Input: part model. Units: mm. Frame: model coordinates. Face numbers are marked on the shaded views. A direction names the side the tool comes from. Round coordinates to 2 decimals unless told otherwise and drop trailing zeros. Loops run counter-clockwise (first coordinate to the right, second up) from the corner with the lowest first, then second, coordinate; pieces in that order, holes last. Notation, with made-up numbers: M -3,3 L 46,3 A11 ccw 46,19 Z; hole C -35,58 d3. An arc over 180 degrees is marked long. Return JSON: item names as keys, results as strings. Group by question number.
1) Access query for the marked faces 1, 2, 3, 4 and 5. Directions: +Z, -Z, +X, -X, +Y, -Y. A direction counts if a zero-diameter tool reaches every point of the face in a straight line with its end or side. Return the directions, or none.
2) Contact query for flat-ended pins moving along their axis: P1, Ø1, axis at y = 11, z = 55, coming from the +X side; P2, Ø14, axis at x = 61.5, z = 40.5, coming from the +Y side; P3, Ø6, axis at x = -3.5, z = 52.5, coming from the -Y side. Output: stop coordinate, or through.
3) Section D-D (y = 37). Output: boundary loops of the cut face in (x, z).
4) Mould query, pull axis Z, two halves, no side actions, for the marked faces 6, 7, 8 and 9. Classes: +Z half, -Z half, draft (parallel to the pull), parting line (faces both ways), or undercut.
5) Section C-C (x = -2.5). Output: boundary loops of the cut face in (y, z).
6) Material intervals for line 1 (X direction, y = 12, z = 53); line 2 (Y direction, x = -45, z = 59); line 3 (Z direction, x = 63, y = 21.5), sorted ascending. Write a range as from..to.
7) Section A-A (z = 75.5). Output: boundary loops of the cut face in (x, y), plus the area to 3 significant figures.
8) Section B-B (x = 45). Output: boundary loops of the cut face in (y, z), plus the area to 3 significant figures.
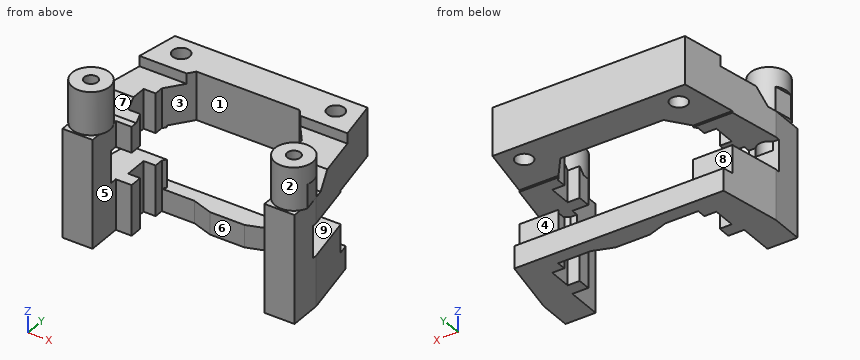
from build123d import *

# Parameters (mm, degrees)
SZKIC1_W                        = 1
SZKIC1_H                        = 32
DODANIE_WYCI_GNI_CIE1_DEPTH     = 67.5
WYTNIJ_WYCI_GNI_CIE1_DEPTH      = 94
WYTNIJ_WYCI_GNI_CIE2_DEPTH      = 36
WYTNIJ_WYCI_GNI_CIE2_DEPTH_BACK = 135
WYTNIJ_WYCI_GNI_CIE6_REACH      = 131.943
SZKIC6_R                        = 5
SZKIC7_R                        = 6.5
WYTNIJ_WYCI_GNI_CIE7_DEPTH      = 20
SZKIC8_R                        = 11
SZKIC8_R_2                      = 3.9
DODANIE_WYCI_GNI_CIE2_DEPTH     = 25
WYTNIJ_WYCI_GNI_CIE8_DEPTH      = 94


with BuildPart() as part:
    # Szkic1 → Dodanie-wyciągnięcie1 (new, symmetric)
    with BuildSketch(Plane(origin=(0, 0, 0), x_dir=(0, 0, -1), z_dir=(1, 0, 0))):
        Polygon((-63, 24), (-71, 32), (-71, 56), (-77, 56), (-77, 80), (-49, 80), (-49, 16), (-29.3, 16), (-29.3, 48), (-13, 48), (-13, 54), (0, 54), (0, 0), (-63, 0), align=None)
        with Locations((-48.5, 32)):
            Rectangle(SZKIC1_W, SZKIC1_H)
    extrude(amount=DODANIE_WYCI_GNI_CIE1_DEPTH, both=True)

    # Szkic2 → Wytnij-wyciągnięcie1 (cut)
    with BuildSketch(Plane(origin=(0, 0, 0), x_dir=(-1, 0, 0), z_dir=(0, 0, -1))):
        Polygon((50, 0), (50, 20), (40.75, 20), (40.75, 27.4), (47.75, 27.4), (47.75, 40.7), (40.75, 40.7), (40.75, 46), (21.75, 46), (10, 42), (-10, 42), (-21.75, 46), (-40.75, 46), (-40.75, 40.7), (-47.75, 40.7), (-47.75, 27.4), (-40.75, 27.4), (-40.75, 20), (-50, 20), (-50, 0), align=None)
    extrude(amount=-WYTNIJ_WYCI_GNI_CIE1_DEPTH, mode=Mode.SUBTRACT)

    # Szkic4 → Wytnij-wyciągnięcie2 (cut, two sides: drawn at the far end of the back side and taken through both)
    with BuildSketch(Plane(origin=(0, 0, 49), x_dir=(-1, 0, 0), z_dir=(0, 0, -1)).offset(-WYTNIJ_WYCI_GNI_CIE2_DEPTH_BACK)):
        Polygon((40.75, 40.7), (40.75, 46), (30, 60), (-30, 60), (-40.75, 46), (-40.75, 40.7), align=None)
    extrude(amount=WYTNIJ_WYCI_GNI_CIE2_DEPTH + WYTNIJ_WYCI_GNI_CIE2_DEPTH_BACK, mode=Mode.SUBTRACT)

    # Szkic6 → Wytnij-wyciągnięcie6 (cut, up to next)
    with BuildSketch(Plane.XY.offset(77), mode=Mode.PRIVATE) as wytnij_wyci_gni_cie6_sk1:
        with Locations((-45, 69)):
            Circle(SZKIC6_R)
    wytnij_wyci_gni_cie6_tool1 = extrude(wytnij_wyci_gni_cie6_sk1.sketch, amount=-WYTNIJ_WYCI_GNI_CIE6_REACH, mode=Mode.PRIVATE) & part.part
    # Szkic6 → Wytnij-wyciągnięcie6 (cut, up to next)
    with BuildSketch(Plane.XY.offset(77), mode=Mode.PRIVATE) as wytnij_wyci_gni_cie6_sk2:
        with Locations(Location((45, 69, 0), (0, 0, 270))):
            Circle(SZKIC6_R)
    wytnij_wyci_gni_cie6_tool2 = extrude(wytnij_wyci_gni_cie6_sk2.sketch, amount=-WYTNIJ_WYCI_GNI_CIE6_REACH, mode=Mode.PRIVATE) & part.part
    add(wytnij_wyci_gni_cie6_tool1.solids().sort_by_distance((-45, 69, 77))[0], mode=Mode.SUBTRACT)
    add(wytnij_wyci_gni_cie6_tool2.solids().sort_by_distance((45, 69, 77))[0], mode=Mode.SUBTRACT)

    # Szkic7 → Wytnij-wyciągnięcie7 (cut)
    with BuildSketch(Plane.XY.offset(63)):
        with Locations((-59, 12)):
            Circle(SZKIC7_R)
        with Locations(Location((59, 12, 0), (0, 0, 37.979872445))):
            Circle(SZKIC7_R)
    extrude(amount=-WYTNIJ_WYCI_GNI_CIE7_DEPTH, mode=Mode.SUBTRACT)

    # Szkic8 → Dodanie-wyciągnięcie2 (add)
    # profile 1 of 2: a face of its own
    with BuildSketch(Plane.XY.offset(63)):
        with Locations(Location((-59, 12, 0), (0, 0, 219.400568754))):
            Circle(SZKIC8_R)
        with Locations((-59, 12)):
            Circle(SZKIC8_R_2, mode=Mode.SUBTRACT)
    # profile 2 of 2: a face of its own
    with BuildSketch(Plane.XY.offset(63)):
        with Locations(Location((59, 12, 0), (0, 0, 180))):
            Circle(SZKIC8_R)
        with Locations(Location((59, 12, 0), (0, 0, 180))):
            Circle(SZKIC8_R_2, mode=Mode.SUBTRACT)
    extrude(amount=DODANIE_WYCI_GNI_CIE2_DEPTH)

    # Szkic9 → Wytnij-wyciągnięcie8 (cut)
    with BuildSketch(Plane.XY.offset(77)):
        Polygon((-71, 0), (-56, 80), (56, 80), (71, 0), (104.197926063, 0), (104.197926063, 108.650562656), (-104.197926063, 108.650562656), (-104.197926063, 0), align=None)
    extrude(amount=-WYTNIJ_WYCI_GNI_CIE8_DEPTH, mode=Mode.SUBTRACT)


solid = part.part
Returned:
{
 "1": {"face 1": "+Z, -Z, -Y", "face 2": "+Z", "face 3": "+Z, -Y", "face 4": "+X, -X, +Y", "face 5": "-Z, -Y"},
 "2": {"P1": "stops at x = 67.5", "P2": "stops at y = 16", "P3": "stops at y = 60"},
 "3": {"outline": "M -64.06,0 L -47.75,0 L -47.75,29.3 L -64.06,29.3 Z; M -64.06,48 L -47.75,48 L -47.75,71 L -64.06,71 Z; M 47.75,0 L 64.06,0 L 64.06,29.3 L 47.75,29.3 Z; M 47.75,48 L 64.06,48 L 64.06,71 L 47.75,71 Z"},
 "4": {"face 6": "draft", "face 7": "+Z half", "face 8": "undercut", "face 9": "undercut"},
 "5": {"outline": "M 42,0 L 54,0 L 54,13 L 42,13 Z; M 60,49 L 80,49 L 80,77 L 60,77 Z"},
 "6": {"line 1": "x = -67.5..-65.5, -52.5..-50, 50..52.5, 65.5..67.5", "line 2": "y = 20..27.4, 40.7..64, 74..80", "line 3": "z = 0..29.3, 48..88"},
 "7": {"outline": "M -69.41,8.46 A11 ccw long -67.42,19.07 Z; M -60.5,56 L -33.07,56 L -30,60 L 30,60 L 33.07,56 L 60.5,56 L 56,80 L -56,80 Z; M 67.42,19.07 A11 ccw long 69.41,8.46 Z; hole C -59,12 d7.8; hole C -45,69 d10; hole C 45,69 d10; hole C 59,12 d7.8", "area": "3,030 mm^2"},
 "8": {"outline": "M 20,0 L 27.4,0 L 27.4,29.3 L 20,29.3 Z; M 20,48 L 27.4,48 L 27.4,66.4 L 24,63 L 20,63 Z; M 40.7,0 L 54,0 L 54,13 L 48,13 L 48,29.3 L 40.7,29.3 Z; M 40.7,48 L 48,48 L 48,49 L 64,49 L 64,77 L 56,77 L 56,71 L 40.7,71 Z; M 74,49 L 80,49 L 80,77 L 74,77 Z", "area": "1,360 mm^2"}
}
